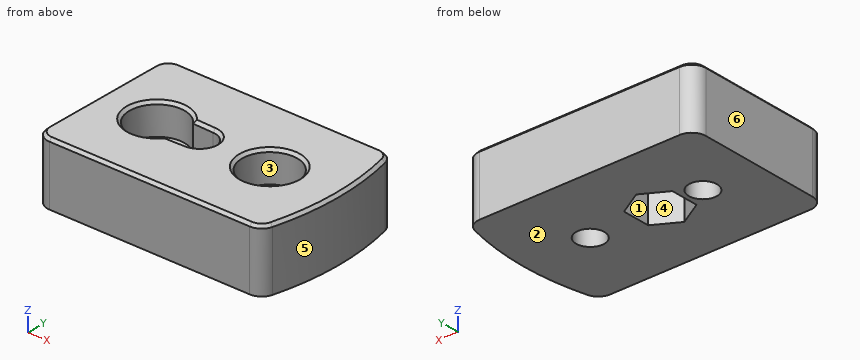
from build123d import *

# Parameters (mm, degrees)
BOSS_EXTRUDE1_DEPTH     = 11
SKETCH2_R               = 2.5
CUT_EXTRUDE1_DEPTH      = 29.018788339
SKETCH3_R               = 4.875
CUT_EXTRUDE2_DEPTH      = 5.5
SKETCH4_R               = 2.75
CUT_EXTRUDE3_DEPTH      = 29.018788339
CUT_EXTRUDE4_DEPTH      = 5.5
FILLET1_R               = 2.5
CHAMFER1_SIZE           = 0.5
CUT_EXTRUDE5_DEPTH      = 29.018788339
CUT_EXTRUDE5_DEPTH_BACK = 29.018788339
CHAMFER3_SIZE           = 0.5


with BuildPart() as part:
    # Sketch1 → Boss-Extrude1 (new body)
    with BuildSketch(Plane.XY):
        with BuildLine():
            Line((-20, -13.5), (20, -13.5))
            ThreePointArc((20, -13.5), (21.95, 0), (20, 13.5))
            Line((20, 13.5), (-20, 13.5))
            Line((-20, 13.5), (-20, -13.5))
        make_face()
    extrude(amount=BOSS_EXTRUDE1_DEPTH)

    # Sketch2 → Cut-Extrude1 (cut, through all)
    with BuildSketch(Plane.XY.offset(11)):
        with Locations((-10, 0)):
            Circle(SKETCH2_R)
        with Locations((10.026646142, 0)):
            Circle(SKETCH2_R)
    extrude(amount=-CUT_EXTRUDE1_DEPTH, mode=Mode.SUBTRACT)

    # Sketch3 → Cut-Extrude2 (cut)
    with BuildSketch(Plane.XY.offset(11)):
        with Locations((-10, 0)):
            Circle(SKETCH3_R)
        with Locations((10.026646142, 0)):
            Circle(SKETCH3_R)
    extrude(amount=-CUT_EXTRUDE2_DEPTH, mode=Mode.SUBTRACT)

    # Sketch4 → Cut-Extrude3 (cut, through all)
    with BuildSketch(Plane.XY.offset(11)):
        with Locations((-2.42, 0)):
            Circle(SKETCH4_R)
    extrude(amount=-CUT_EXTRUDE3_DEPTH, mode=Mode.SUBTRACT)

    # Sketch5 → Cut-Extrude4 (cut)
    with BuildSketch(Plane(origin=(0, 0, 0), x_dir=(-1, 0, 0), z_dir=(0, 0, -1))):
        Polygon((6.72, -2.482606158), (6.72, 2.482606158), (2.42, 4.965212315), (-1.88, 2.482606158), (-1.88, -2.482606158), (2.42, -4.965212315), align=None)
    extrude(amount=-CUT_EXTRUDE4_DEPTH, mode=Mode.SUBTRACT)

    # Fillet1
    fillet1_edges = [part.edges().sort_by_distance(p)[0] for p in [
        (20, -13.5, 5.5),
        (-20, -13.5, 5.5),
        (-20, 13.5, 5.5),
        (20, 13.5, 5.5),
    ]]
    fillet(fillet1_edges, radius=FILLET1_R)

    # Chamfer1
    chamfer1_edges = [part.edges().sort_by_distance(p)[0] for p in [
        (0.295627716, -13.5, 11),
        (-20, 0, 11),
        (21.95, 0, 11),
        (0.295627716, 13.5, 11),
        (19.628977191, 12.971144792, 11),
        (19.628977191, -12.971144792, 11),
        (-19.267766953, 12.767766953, 11),
        (-19.267766953, -12.767766953, 11),
    ]]
    chamfer(chamfer1_edges, length=CHAMFER1_SIZE)

    # Sketch6 → Cut-Extrude5 (cut, two sides: drawn at the far end of the back side and taken through both)
    with BuildSketch(Plane.XY.offset(11).offset(-CUT_EXTRUDE5_DEPTH_BACK)):
        with BuildLine():
            Line((-6.05629261, 2.865797798), (-2.42, 2.75))
            ThreePointArc((-2.42, 2.75), (0.33, 0), (-2.42, -2.75))
            Line((-2.42, -2.75), (-6.05629261, -2.865797798))
            Line((-6.05629261, -2.865797798), (-6.72, -2.482606158))
            Line((-6.72, -2.482606158), (-6.72, 2.482606158))
            Line((-6.72, 2.482606158), (-6.05629261, 2.865797798))
        make_face()
    extrude(amount=CUT_EXTRUDE5_DEPTH + CUT_EXTRUDE5_DEPTH_BACK, mode=Mode.SUBTRACT)

    # Chamfer3
    chamfer3_edges = [part.edges().sort_by_distance(p)[0] for p in [
        (0.33, 0, 11),
        (-14.875, 0, 11),
        (-4.238146305, 2.807898899, 11),
        (-4.238146305, -2.807898899, 11),
        (5.151646142, 0, 11),
    ]]
    chamfer(chamfer3_edges, length=CHAMFER3_SIZE)


solid = part.part
Here's how the part is built. I have some questions about the finished solid (model axes, mm). Face numbers are marked on the shaded views. A direction names the side the tool comes from. Round coordinates to 2 decimals unless told otherwise and drop trailing zeros. Loops run counter-clockwise (first coordinate to the right, second up) from the corner with the lowest first, then second, coordinate; pieces in that order, holes last.
1. If we section it at B-B on y = 0: Count the separate pieces of the cut face and the enclosed holes in it, plus the area to 3 significant figures.
Answer list:
separate pieces: 4
enclosed holes: 0
area: 221 mm2
2. If I drill on line 1 along Y through (x, z) = (-10, 4.1); line 2 along Y through (x, z) = (-10, 8) (3 decimals); line 3 along Z through (x, y) = (8, 2.75), over which ranges is the centre line in solid material (lowest first)?
Answer list:
line 1: y = -13.5 to -2.5, 2.5 to 13.5
line 2: y = -13.5 to -4.875, 4.875 to 13.5
line 3: z = 0 to 5.5
3. If we section it at A-A on x = -10: Write out the boundary of the cut face in (y, z) (3 decimals).
Answer list:
outline: (-13.5, 0) - (-2.5, 0) - (-2.5, 5.5) - (-4.875, 5.5) - (-4.875, 10.5) - (-5.375, 11) - (-13, 11) - (-13.5, 10.5) - close; (2.5, 0) - (13.5, 0) - (13.5, 10.5) - (13, 11) - (5.375, 11) - (4.875, 10.5) - (4.875, 5.5) - (2.5, 5.5) - close
4. Which directions (+Z, -Z, +X, -X, +Y, -Y) give clear straight access to the entire face, cutting with the end or side of a thin tool? Please do the marked faces 1, 2 and 3.
Answer list:
face 1: -Z
face 2: -Z, +X, -X, +Y, -Y
face 3: +Z
5. We'd pull the mould along X, two halves only. Please class the marked faces 4, 5 and 6: +X half, -X half, draft (parallel to the pull), parting line (faces both ways), or undercut.
Answer list:
face 4: undercut
face 5: +X half
face 6: -X half
6. If we section it at D-D on z = 9.75: Write out the boundary of the cut face in (x, y) (3 decimals).
Answer list:
outline: (-20, -11) arc R2.5 ccw to (-17.5, -13.5) - (18.091, -13.5) arc R2.5 ccw to (20.516, -11.608) arc R47.706 ccw to (20.516, 11.608) arc R2.5 ccw to (18.091, 13.5) - (-17.5, 13.5) arc R2.5 ccw to (-20, 11) - close; hole (-6.056, -2.866) - (-2.42, -2.75) arc R2.75 ccw to (-2.42, 2.75) - (-6.056, 2.866) arc R4.875 ccw (long way) to start; hole circle Ø9.75 at (10.027, 0)
7. If we section it at C-C on z = 2.5: Write out the boundary of the cut face in (x, y), plus the area to 3 significant figures.
Answer list:
outline: (-20, -11) arc R2.5 ccw to (-17.5, -13.5) - (18.09, -13.5) arc R2.5 ccw to (20.52, -11.61) arc R47.71 ccw to (20.52, 11.61) arc R2.5 ccw to (18.09, 13.5) - (-17.5, 13.5) arc R2.5 ccw to (-20, 11) - close; hole circle Ø5 at (-10, 0); hole (-6.72, -2.48) - (-2.42, -4.97) - (1.88, -2.48) - (1.88, 2.48) - (-2.42, 4.97) - (-6.72, 2.48) - close; hole circle Ø5 at (10.03, 0)
area: 1,010 mm2
8. For P1, Ø6, axis at y = 8, z = 8, coming from the +X side; P2, Ø5, axis at x = 9, y = 1, coming from the +Z side; P3, Ø4.5, axis at x = 10.03, y = 0, coming from the -Z side, each with a flat end and sliding along its axis, tell me the tip position at first contact or that it passes through.
Answer list:
P1: stops at x = 21.69
P2: stops at z = 5.5
P3: passes through
